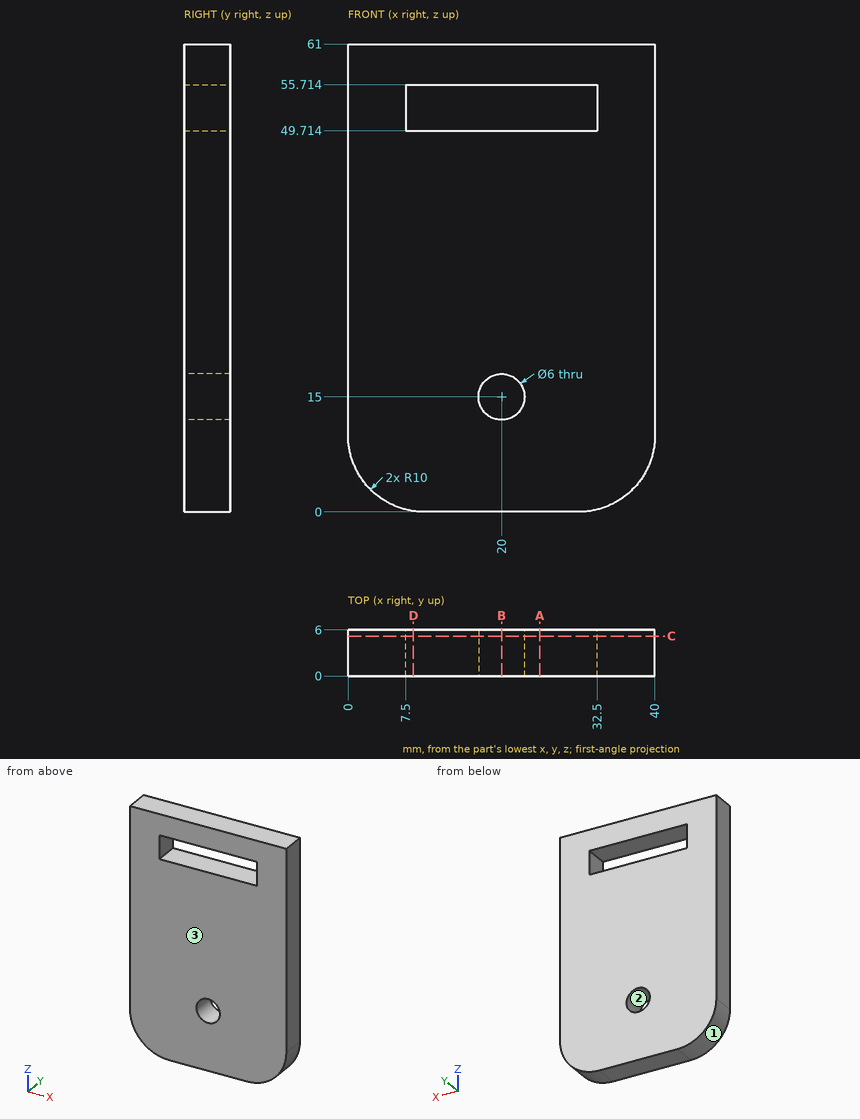
Geometry check sheet. Reference: drawing and pictorial views, mm from the part's lowest x, y, z. Give positions to 0.01 mm unless a question says otherwise; leave off trailing zeros. Order: outer loops, then holes, each group sorted by start corner. A loop starts at its lowest first (then second) coordinate and runs counter-clockwise, first axis right, second up. Notation, with made-up numbers: M 50,-23 L 101,-23 A24 ccw 101,-1 Z; hole C 1.25,66 d2. An arc over 180 degrees is marked long. Answer in a Markdown table with one row per item.
1) Thickness scan on L1, parallel to Z at x = 20, y = 2.4; L2, parallel to X at y = 1.5, z = 15; L3, parallel to X at y = 3, z = 55. Record the ranges inside material, lowest first. Write a range as [from, to].
Filled sheet:
| item | result |
|---|---|
| L1 | z = [0, 12], [18, 49.71], [55.71, 61] |
| L2 | x = [0, 17], [23, 40] |
| L3 | x = [0, 7.5], [32.5, 40] |
2) Cross-section at A-A, the plane x = 25. Enter the section's corners in (y, z).
Filled sheet:
| item | result |
|---|---|
| outline | M 0,0 L 6,0 L 6,49.71 L 0,49.71 Z; M 0,55.71 L 6,55.71 L 6,61 L 0,61 Z |
3) Cross-section at B-B, the plane x = 20. Enter the section's corners in (y, z).
Filled sheet:
| item | result |
|---|---|
| outline | M 0,0 L 6,0 L 6,12 L 0,12 Z; M 0,18 L 6,18 L 6,49.71 L 0,49.71 Z; M 0,55.71 L 6,55.71 L 6,61 L 0,61 Z |
4) Gauge pin test, flat ends, axial feed: P1, Ø1, axis at x = 32, y = 1.5, coming from the -Z side; P2, Ø1, axis at x = 7.5, y = 2, coming from the -Z side. Record the tip position at first contact, or that the pin passes through.
Filled sheet:
| item | result |
|---|---|
| P1 | stops at z = 0.11 |
| P2 | stops at z = 0.2 |
5) Cross-section at D-D, the plane x = 8.5. Enter the section's corners in (y, z).
Filled sheet:
| item | result |
|---|---|
| outline | M 0,0.11 L 6,0.11 L 6,49.71 L 0,49.71 Z; M 0,55.71 L 6,55.71 L 6,61 L 0,61 Z |
6) Release check for a two-part mould opening along X. For the marked faces 1, 2 and 3 record: +X half, -X half, draft (parallel to the pull), parting line (faces both ways), or undercut.
Filled sheet:
| item | result |
|---|---|
| face 1 | -X half |
| face 2 | undercut |
| face 3 | draft |
7) Cross-section at C-C, the plane y = 5.2. Enter the section's corners in (x, z).
Filled sheet:
| item | result |
|---|---|
| outline | M 0,10 A10 ccw 10,0 L 30,0 A10 ccw 40,10 L 40,61 L 0,61 Z; hole M 7.5,49.71 L 32.5,49.71 L 32.5,55.71 L 7.5,55.71 Z; hole C 20,15 d6 |
